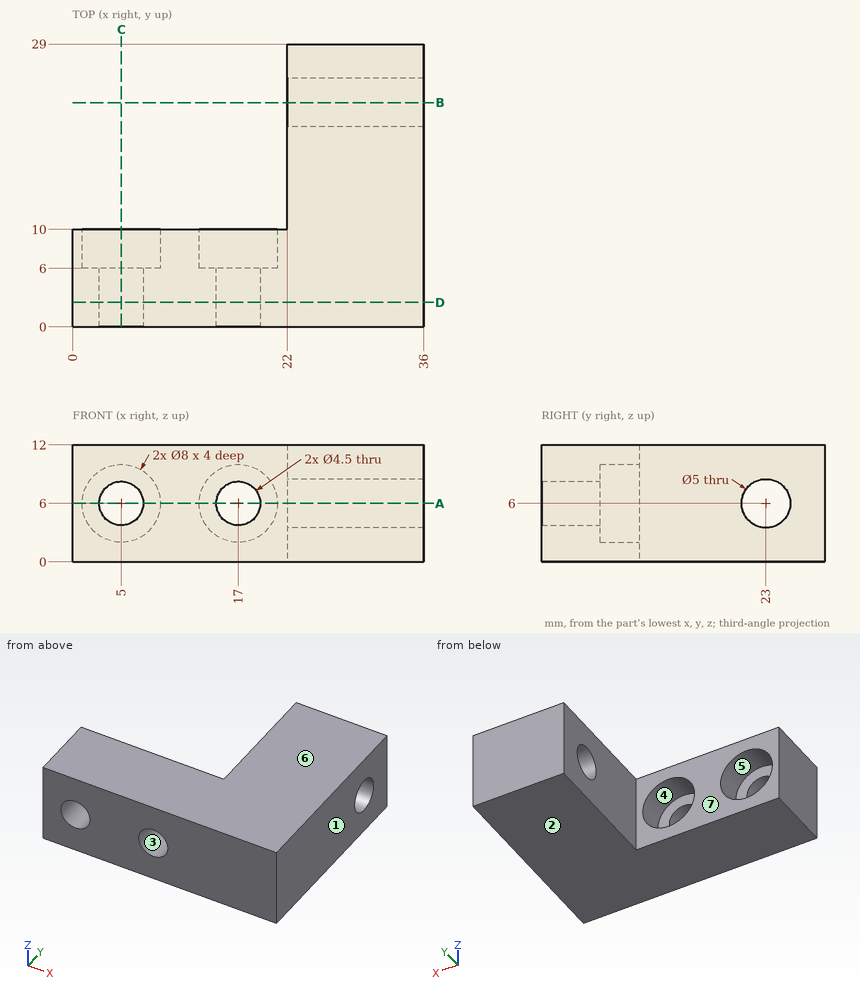
Verification items for this drawing (mm, ordinates from the low corner). A direction names the side the tool comes from. Round coordinates to 2 decimals unless told otherwise and drop trailing zeros. Loops run counter-clockwise (first coordinate to the right, second up) from the corner with the lowest first, then second, coordinate; pieces in that order, holes last. Notation, with made-up numbers: (63.25, -18) - (95.25, -18) arc R17 ccw to (95.25, 13) - close; hole circle Ø10 at (-9, -27.75). An arc over 180 degrees is marked (long way). Write item = value, one per line.
Q1. Tool access check on the marked faces 5, 6 and 7. Record the directions out of +Z, -Z, +X, -X, +Y, -Y that give a thin tool (end or side, any length) a straight path to the whole face; none if there is none.
Here are the results:
face_5 = +Y
face_6 = +Z, +X, -X, +Y, -Y
face_7 = +Z, -Z, -X, +Y
Q2. Material ranges on L1, parallel to X at y = 4.5, z = 6; L2, parallel to X at y = 8.25, z = 5.75; L3, parallel to Z at x = 17, y = 8.3, recorded low to high.
Here are the results:
L1 = 0 to 2.75, 7.25 to 14.75, 19.25 to 36
L2 = 0 to 1.01, 8.99 to 13.01, 20.99 to 36
L3 = 0 to 2, 10 to 12
Q3. Depth check by flat-ended pin: pin 1 (6 mm diameter, centred on y = 20.5, z = 9.5, fed in from -X); pin 2 (6 mm diameter, centred on x = 8.5, z = 3.5, fed in from +Y); pin 3 (6.5 mm diameter, centred on x = 17, z = 6, fed in from +Y); pin 4 (2.5 mm diameter, centred on x = 17, z = 6, fed in from -Y). Enter the tip coordinate at first touch or a pass-through.
Here are the results:
pin_1 = 22
pin_2 = 10
pin_3 = 6
pin_4 = through
Q4. Sectioned sample at A-A on z = 6. Record the boundary of the cut face in (x, y), plus the area to 3 significant figures.
Here are the results:
outline = (0, 0) - (2.75, 0) - (2.75, 6) - (1, 6) - (1, 10) - (0, 10) - close; (7.25, 0) - (14.75, 0) - (14.75, 6) - (13, 6) - (13, 10) - (9, 10) - (9, 6) - (7.25, 6) - close; (19.25, 0) - (36, 0) - (36, 20.5) - (22, 20.5) - (22, 10) - (21, 10) - (21, 6) - (19.25, 6) - close; (22, 25.5) - (36, 25.5) - (36, 29) - (22, 29) - close
area = 438 mm^2
Q5. Mould release check, pull along X, two halves, no side actions. Record for the marked faces 1, 2, 3 and 4: +X half, -X half, draft (parallel to the pull), parting line (faces both ways), or undercut.
Here are the results:
face_1 = +X half
face_2 = draft
face_3 = undercut
face_4 = undercut
Q6. Sectioned sample at C-C on x = 5. Record the boundary of the cut face in (y, z), plus the area to 3 significant figures.
Here are the results:
outline = (0, 0) - (10, 0) - (10, 2) - (6, 2) - (6, 3.75) - (0, 3.75) - close; (0, 8.25) - (6, 8.25) - (6, 10) - (10, 10) - (10, 12) - (0, 12) - close
area = 61.0 mm^2
Q7. Sectioned sample at D-D on y = 2.5. Record the boundary of the cut face in (x, z).
Here are the results:
outline = (0, 0) - (36, 0) - (36, 12) - (0, 12) - close; hole circle Ø4.5 at (5, 6); hole circle Ø4.5 at (17, 6)
Q8. Sectioned sample at B-B on y = 23. Record the boundary of the cut face in (x, z).
Here are the results:
outline = (22, 0) - (36, 0) - (36, 3.5) - (22, 3.5) - close; (22, 8.5) - (36, 8.5) - (36, 12) - (22, 12) - close
